Check sheet for the modelled part. Datum: model origin and axes. Units: mm. A direction names the side the tool comes from. Round coordinates to 2 decimals unless told otherwise and drop trailing zeros. Loops run counter-clockwise (first coordinate to the right, second up) from the corner with the lowest first, then second, coordinate; pieces in that order, holes last. Notation, with made-up numbers: (54, -36) - (95, -36) arc R15 cw to (95, -8) - close; hole circle Ø5 at (-17, 79). An arc over 180 degrees is marked (long way). Return JSON: item names as keys, results as strings.
from build123d import *

# Parameters (mm, degrees)
F0_W     = 30.48
F0_H     = 9.525
F1_DEPTH = 7.62
F2_R     = 3.175
F2_R_2   = 2.54
F3_DEPTH = 0.762
F4_DEPTH = 10.16
F5_R     = 2.413
F5_R_2   = 1.5875
F6_DEPTH = 1.905


with BuildPart() as f1:
    # F0 (on Front) → F1 (new body)
    with BuildSketch(Plane.XZ):
        with Locations((15.24, 4.7625)):
            Rectangle(F0_W, F0_H)
    extrude(amount=-F1_DEPTH)

    # F2 (on face) → F3 (cut)
    with BuildSketch(Plane.XZ):
        with Locations((7.62, 5.715)):
            Circle(F2_R)
        with Locations((7.62, 5.715)):
            Circle(F2_R_2, mode=Mode.SUBTRACT)
        with Locations((15.24, 5.715)):
            Circle(F2_R)
        with Locations((15.24, 5.715)):
            Circle(F2_R_2, mode=Mode.SUBTRACT)
        with Locations((22.86, 5.715)):
            Circle(F2_R)
        with Locations((22.86, 5.715)):
            Circle(F2_R_2, mode=Mode.SUBTRACT)
    extrude(amount=-F3_DEPTH, mode=Mode.SUBTRACT)

    # F4 (cut): faces of the model
    f4_faces = [f1.faces().sort_by_distance(p)[0] for p in [
        (7.62, 0, 5.715),
        (15.24, 0, 5.715),
        (22.86, 0, 5.715),
    ]]
    extrude(f4_faces, amount=-F4_DEPTH, mode=Mode.SUBTRACT)

    # F5 (on face) → F6 (join)
    with BuildSketch(Plane.XY.offset(9.525)):
        with Locations((3.81, 3.7642538082)):
            Circle(F5_R)
        with Locations((3.81, 3.7642538082)):
            Circle(F5_R_2, mode=Mode.SUBTRACT)
        with Locations((11.43, 3.7592)):
            Circle(F5_R)
        with Locations((11.43, 3.7592)):
            Circle(F5_R_2, mode=Mode.SUBTRACT)
        with Locations((19.05, 3.7541461918)):
            Circle(F5_R)
        with Locations((19.05, 3.7541461918)):
            Circle(F5_R_2, mode=Mode.SUBTRACT)
        with Locations((26.67, 3.81)):
            Circle(F5_R)
        with Locations((26.67, 3.81)):
            Circle(F5_R_2, mode=Mode.SUBTRACT)
    extrude(amount=F6_DEPTH)


solid = f1.part
Q1. Sectioned sample at A-A (x = 22.86). Enter the section's corners in (y, z) (3 decimals).
Answer key:
{"outline": "(0, 0) - (7.62, 0) - (7.62, 3.175) - (0.762, 3.175) - (0.762, 2.54) - (0, 2.54) - close; (0, 8.89) - (0.762, 8.89) - (0.762, 8.255) - (7.62, 8.255) - (7.62, 9.525) - (0, 9.525) - close"}
Q2. Sectioned sample at B-B (z = 10.5). State how many separate pieces and enclosed holes the cut face has, plus the area to 3 significant figures.
Answer key:
{"separate pieces": "4", "enclosed holes": "4", "area": "41.5 mm²"}
Q3. Sectioned sample at C-C (z = 7). Enter the section's corners in (x, y), plus the area to 3 significant figures.
Answer key:
{"outline": "(0, 0) - (4.72, 0) - (4.72, 0.76) - (5.43, 0.76) - (5.43, 7.62) - (0, 7.62) - close; (9.81, 0.76) - (10.52, 0.76) - (10.52, 0) - (12.34, 0) - (12.34, 0.76) - (13.05, 0.76) - (13.05, 7.62) - (9.81, 7.62) - close; (17.43, 0.76) - (18.14, 0.76) - (18.14, 0) - (19.96, 0) - (19.96, 0.76) - (20.67, 0.76) - (20.67, 7.62) - (17.43, 7.62) - close; (25.05, 0.76) - (25.76, 0.76) - (25.76, 0) - (30.48, 0) - (30.48, 7.62) - (25.05, 7.62) - close", "area": "129 mm²"}
Q4. Depth check by flat-ended pin: P1, Ø1.5, axis at x = 15, y = 5, coming from the -Z side; P2, Ø3, axis at x = 26.67, y = 3.81, coming from the +Z side (3 decimals); P3, Ø5, axis at x = 22.86, z = 5.715, coming from the -Y side (1 decimal). Enter the tip coordinate at first touch or a pass-through.
Answer key:
{"P1": "stops at z = 0", "P2": "stops at z = 9.525", "P3": "passes through"}
Q5. Tool access check on faces 1 (the face through (15, 4, 0)), 2 (the face through (11.116, 6.152, 10.464)), 3 (the face through (12.72, 0.376, 3.783)). Record the directions out of +Z, -Z, +X, -X, +Y, -Y that give a thin tool (end or side, any length) a straight path to the whole face; none if there is none.
Answer key:
{"face 1": "-Z, +X, -X, +Y, -Y", "face 2": "+Z", "face 3": "-Y"}
Q6. Sectioned sample at D-D (x = 3.81). Enter the section's corners in (y, z) (3 decimals), plus the area to 3 significant figures.
Answer key:
{"outline": "(0, 0) - (7.62, 0) - (7.62, 9.525) - (6.177, 9.525) - (6.177, 11.43) - (5.352, 11.43) - (5.352, 9.525) - (2.177, 9.525) - (2.177, 11.43) - (1.351, 11.43) - (1.351, 9.525) - (0, 9.525) - close", "area": "75.7 mm²"}
Q7. Draft check along Z on faces 4 (the face through (15, 0, 2)), 5 (the face through (4, 4, 9.525)), 6 (the face through (20.844, 4.143, 4.169)). Enter one of: released by +Z, released by -Z, zero draft, split by the parting line, or undercut.
Answer key:
{"face 4": "zero draft", "face 5": "released by +Z", "face 6": "undercut"}
Q8. Scan lines: probe 1 along Z at (x, y) = (15.24, 5.5) (3 decimals); probe 2 along Y at (x, z) = (3.81, 11.05); probe 3 along X at (y, z) = (5.75, 3.75). Record each from-to range of solid material in increasing order. Write a range as [from, to].
Answer key:
{"probe 1": "z = [0, 3.175], [8.255, 9.525]", "probe 2": "y = [1.35, 2.18], [5.35, 6.18]", "probe 3": "x = [0, 6.01], [9.23, 13.63], [16.85, 21.25], [24.47, 30.48]"}
